Geometry check sheet. Reference: the model listing, model coordinates, mm. Face numbers are marked on the shaded views. Round coordinates to 2 decimals unless told otherwise and drop trailing zeros. Order: outer loops, then holes, each group sorted by start corner. A loop starts at its lowest first (then second) coordinate and runs counter-clockwise, first axis right, second up.
(1) Draft check along X on the marked faces 1, 2 and 3. Enter one of: pulls with the +X half, pulls with the -X half, needs draft (parallel to the pull), parting line crosses it, or undercut.
(2) Thickness scan on L1, parallel to Y at x = 0, z = -0.75; L2, parallel to X at y = 0.5, z = -0.25; L3, parallel to Z at x = 5.25, y = -6. Record the ranges inside material, lowest first.
(3) Cross-section at A-A on y = 0. Enter the section's corners in (x, z).
(4) Cross-section at C-C on z = -1.05. Enter the section's corners in (x, y), and give its area (3 significant figures).
(5) Gauge pin test, flat end, axial feed: P1, Ø1, axis at x = -6, z = -1, coming from the +Y side. Record the tip position at first contact, or that the pin passes through.
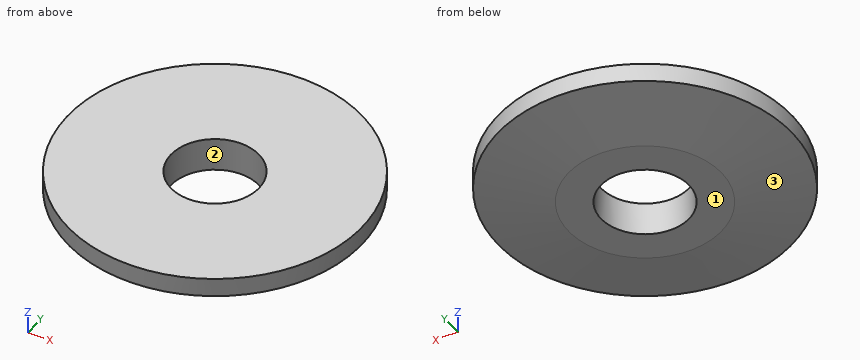
from build123d import *

# Parameters (mm, degrees)
CYLINDER_R                     = 15
CYLINDER_DEPTH                 = 10
REVOLVE_ONTO_SKETCH_ROLL_ANGLE = 90


with BuildPart() as cylinder:
    # Cylinder → Cylinder (new body)
    with BuildSketch(Plane.XY):
        Circle(CYLINDER_R)
    extrude(amount=CYLINDER_DEPTH)


with BuildPart() as cut_float:
    # Sketch as drawn → Revolve (revolve)
    with BuildSketch(Plane.XY):
        Polygon((-3, 0), (-5.213686, 0), (-10, 1), (-10, 5), (-3, 5), align=None)
    revolve(axis=Axis((0, 0, 0), (0, 1, 0)))


with BuildPart() as cut_float_1:
    # Revolve onto Sketch roll: moved
    add(cut_float.part.rotate(Axis((0, 0, 0), (1, 0, 0)), REVOLVE_ONTO_SKETCH_ROLL_ANGLE))


with BuildPart() as cut_float_2:
    # Revolve onto Sketch placement: moved
    add(cut_float_1.part)


with BuildPart() as cut_float_3:
    # Revolve placement: moved
    add(cut_float_2.part.moved(Location((0, 0, -2.28))))

    # Cut: cut Cylinder
    add(cylinder.part, mode=Mode.SUBTRACT)


solid = cut_float_3.part
Found:
1. face 1: needs draft
1. face 2: undercut
1. face 3: parting line crosses it
2. L1: y = -10 to -3, 3 to 10
2. L2: x = -9.99 to -2.96, 2.96 to 9.99
2. L3: z = -1.7 to 0
3. outline: (-10, -1.28) - (-5.21, -2.28) - (-3, -2.28) - (-3, 0) - (-10, 0) - close; (3, -2.28) - (5.21, -2.28) - (10, -1.28) - (10, 0) - (3, 0) - close
4. outline: circle Ø20 at (0, 0); hole circle Ø6 at (0, 0)
4. area: 286 mm2
5. P1: stops at y = 8.35
